from build123d import *

# Parameters (mm, degrees)
SKETCH1_W           = 3.2
SKETCH1_H           = 15
BOSS_EXTRUDE1_DEPTH = 3.2


with BuildPart() as part:
    # Sketch1 → Boss-Extrude1 (new body)
    with BuildSketch(Plane(origin=(0, 0, 0), x_dir=(0, 0, -1), z_dir=(1, 0, 0))):
        Polygon((-10, 42.5), (-30, 42.5), (-30, 39.3), (-50, 39.3), (-50, 42.5), (-70, 42.5), (-70, 39.3), (-87.5, 39.3), (-87.5, 25), (-84.3, 25), (-84.3, 10), (-87.5, 10), (-87.5, -10), (-84.3, -10), (-84.3, -25), (-87.5, -25), (-87.5, -39.3), (-70, -39.3), (-70, -42.5), (-50, -42.5), (-50, -39.3), (-30, -39.3), (-30, -42.5), (-10, -42.5), (-10, -39.3), (10, -39.3), (10, -42.5), (30, -42.5), (30, -39.3), (50, -39.3), (50, -42.5), (70, -42.5), (70, -39.3), (87.5, -39.3), (87.5, -25), (84.3, -25), (84.3, -10), (87.5, -10), (87.5, 10), (84.3, 10), (84.3, 25), (87.5, 25), (87.5, 39.3), (70, 39.3), (70, 42.5), (50, 42.5), (50, 39.3), (30, 39.3), (30, 42.5), (10, 42.5), (10, 39.3), (-10, 39.3), align=None)
        with Locations((-26.6, 16.8)):
            Rectangle(SKETCH1_W, SKETCH1_H, mode=Mode.SUBTRACT)
        with Locations((26.6, 16.8)):
            Rectangle(SKETCH1_W, SKETCH1_H, mode=Mode.SUBTRACT)
    extrude(amount=BOSS_EXTRUDE1_DEPTH)


solid = part.part
Read the model definition and answer for the solid it produces. Units are mm, in the model's axes. A direction names the side the tool comes from. Round coordinates to 2 decimals unless told otherwise and drop trailing zeros. Write each loop counter-clockwise with the first axis right and the second up, starting at its lowest first coordinate (ties: lowest second). Pieces come first, ordered by that corner, then holes.
1. The part is cut by section B-B, the plane x = 0.75. State how many separate pieces and enclosed holes the cut face has, then the cut area to 3 significant figures.
2. The part is cut by section C-C, the plane y = -15. Determine the outline of the cut face in (x, z).
3. Determine the mould class of faces 1 (the face through (2, 17, 28.2)), 2 (the face through (2, 42.5, -20)), 3 (the face through (2, 32, -87.5)) for opening direction Z: pulls with the +Z half, pulls with the -Z half, needs draft (parallel to the pull), parting line crosses it, or undercut.
4. Which of the six approach directions +Z, -Z, +X, -X, +Y, -Y give full straight-line access (tool end or side, diameter ignored) to faces 4 (the face through (2, 39.3, -40)), 5 (the face through (2, -17, 84.3)), 6 (the face through (2, -41, 50)), 7 (the face through (2, 41, -70))?
5. Given pin 1 Ø1 at (x, z) = (1.5, 39.5) entering from -Y; pin 2 Ø3 at (y, z) = (30, 64.5) entering from -X; pin 3 Ø1 at (x, y) = (1.5, -40.5) entering from -Z, each flat-ended and moving along its own axis, determine where each tip first touches the part or whether it passes through.
6. Straight lines are drawn through the part: L1, parallel to Z at x = 2.55, y = 12; L2, parallel to Y at x = 1.45, z = 44; L3, parallel to Z at x = 0.35, y = -14. For each, find the intervals that lie inside material, in ascending order.
7. The part is cut by section A-A, the plane z = -72. Determine the outline of the cut face in (x, y).
Values:
1. separate pieces: 1
1. enclosed holes: 2
1. area: 14,000 mm2
2. outline: (0, -84.3) - (3.2, -84.3) - (3.2, 84.3) - (0, 84.3) - close
3. face 1: undercut
3. face 2: needs draft
3. face 3: pulls with the -Z half
4. face 4: +X, -X, +Y
4. face 5: +Z, +X, -X
4. face 6: +X, -X, -Y
4. face 7: -Z, +X, -X, +Y
5. pin 1: stops at y = -39.3
5. pin 2: stops at x = 0
5. pin 3: stops at z = -70
6. L1: z = -84.3 to -28.2, -25 to 25, 28.2 to 84.3
6. L2: y = -39.3 to 39.3
6. L3: z = -84.3 to 84.3
7. outline: (0, -39.3) - (3.2, -39.3) - (3.2, 39.3) - (0, 39.3) - close
